Study the drawing (mm; zero at the part's minimum x, y, z) and answer. A direction names the side the tool comes from. Coordinates: 2 decimals unless noted, no trailing zeros. Order: outer loops, then holes, each group sorted by start corner. A loop starts at its lowest first (then second) coordinate and runs counter-clockwise, first axis right, second up. Notation, with made-up numbers: M -37.5,46.5 L -28.5,46.5 A16 cw -28.5,54.5 Z; hole C -2,16.5 d10. An arc over 180 degrees is marked long. Use a Markdown table: item, result. Add a question column.
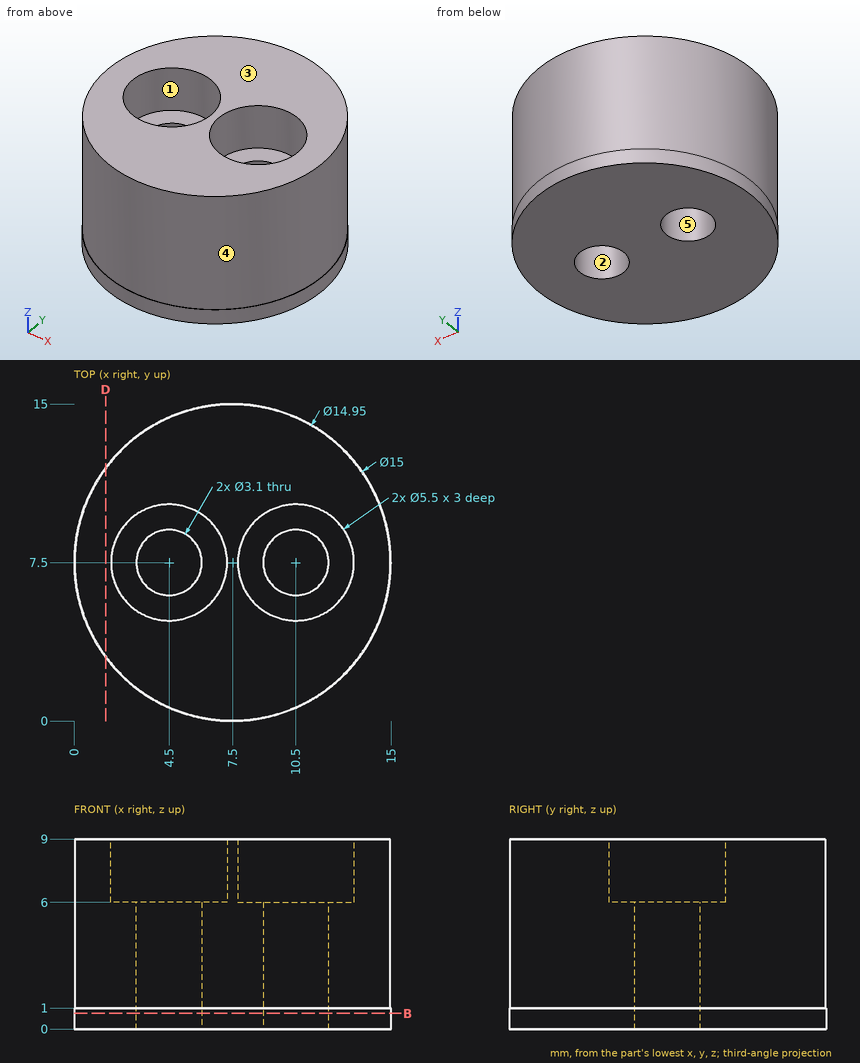
(1) Given P1, Ø1.5, axis at x = 3, z = 1, coming from the +Y side; P2, Ø4, axis at x = 9.5, z = 4.5, coming from the +Y side (3 decimals); P3, Ø1.6, axis at x = 3.5, y = 8, coming from the +Z side; P4, Ø1.9, axis at x = 4.5, y = 7.5, coming from the +Z side, each flat-ended and moving along its own axis, determine where each tip first touches the part or whether it passes through.
(2) Straight lines are drawn through the part: line 1 (X direction, y = 8.75, z = 7.25); line 2 (Z direction, x = 3, y = 6.5); line 3 (X direction, y = 7, z = 2). For each, find the intervals that lie inside material, in ascending order.
(3) A cutting plane is placed at D-D on x = 1.5. Write down the section's boundary in (y, z).
(4) A cutting plane is placed at B-B on z = 0.75. Write down the section's boundary in (x, y).
(5) The mould has two halves that part along X. Classify the marked faces 3, 4 and 5: pulls with the +X half, pulls with the -X half, needs draft (parallel to the pull), parting line crosses it, or undercut.
(6) Which of the six approach directions +Z, -Z, +X, -X, +Y, -Y give full straight-line access (tool end or side, diameter ignored) to the marked faces 1 and 2?
From the geometry:
| question | item | result |
|---|---|---|
| 1 | P1 | stops at y = 14 |
| 1 | P2 | stops at y = 14.975 |
| 1 | P3 | stops at z = 6 |
| 1 | P4 | passes through |
| 2 | line 1 | x = 0.13 to 2.05, 6.95 to 8.05, 12.95 to 14.87 |
| 2 | line 2 | z = 0 to 6 |
| 2 | line 3 | x = 0.04 to 3.03, 5.97 to 9.03, 11.97 to 14.96 |
| 3 | outline | M 3,0 L 12,0 L 12,1 L 11.96,1 L 11.96,9 L 3.04,9 L 3.04,1 L 3,1 Z |
| 4 | outline | C 7.5,7.5 d15; hole C 4.5,7.5 d3.1; hole C 10.5,7.5 d3.1 |
| 5 | face 3 | needs draft |
| 5 | face 4 | parting line crosses it |
| 5 | face 5 | undercut |
| 6 | face 1 | +Z |
| 6 | face 2 | +Z, -Z |
